The figure shows three views and two pictorial views of one solid part (mm, origin at its lowest corner). Answer the questions. A direction names the side the tool comes from. Round coordinates to 2 decimals unless told otherwise and drop trailing zeros. Order: outer loops, then holes, each group sorted by start corner. A loop starts at its lowest first (then second) coordinate and runs counter-clockwise, first axis right, second up. Notation, with made-up numbers: (4, -22) - (48, -22) arc R35 ccw to (48, 16) - close; hole circle Ø2 at (7.25, 42.5). An arc over 180 degrees is marked (long way). One line per item, written item: value. Start each with the question number.
1. Straight lines are drawn through the part: line 1 (X direction, y = 0.4, z = 35); line 2 (Y direction, x = 41, z = 54.5); line 3 (Z direction, x = 27.5, y = 0.85). For each, find the intervals that lie inside material, in ascending order.
2. Section C-C, the plane z = 50.5 is taken. Give the vertices of the cut face in (x, y).
3. Section A-A, the plane x = 7 is taken. Give the vertices of the cut face in (y, z), then the cut area to 3 significant figures.
4. Flat-ended cylindrical pins translate along their axes: P1, Ø0.6, axis at x = 43, y = 1, coming from the -Z side; P2, Ø8, axis at x = 24, z = 48, coming from the +Y side; P3, Ø2, axis at y = 1, z = 15, coming from the +X side. Find the tip coordinate at first contact, or state that the pin passes through.
5. Section B-B, the plane y = 3.5 is taken. Give the vertices of the cut face in (x, z), then the cut area to 3 significant figures.
6. A tool of negligible diameter and unlimited length cuts with its end or side. For the marked faces 1 and 2, from which of +Z, -Z, +X, -X, +Y, -Y can it reach the whole face along a straight path? Write none if from no direction.
7. Section D-D, the plane z = 38 is taken. Give the vertices of the cut face in (x, y).
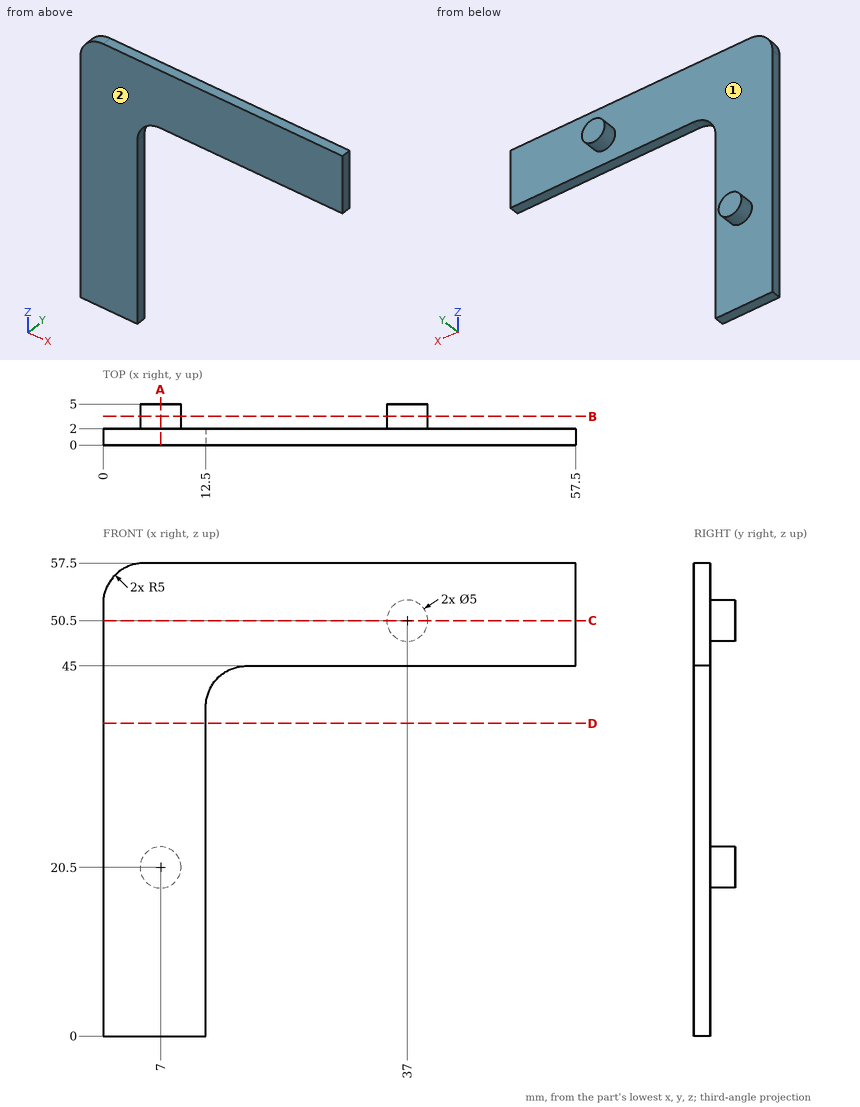
Answer list:
1. line 1: x = 0 to 12.5
1. line 2: y = 0 to 2
1. line 3: z = 45 to 57.5
2. outline: (0, 0) - (57.5, 0) - (57.5, 2) - (39.5, 2) - (39.5, 5) - (34.5, 5) - (34.5, 2) - (0, 2) - close
3. outline: (0, 0) - (2, 0) - (2, 18) - (5, 18) - (5, 23) - (2, 23) - (2, 57.5) - (0, 57.5) - close
3. area: 130 mm²
4. P1: stops at z = 45
4. P2: stops at y = 2
4. P3: stops at x = 12.5
5. outline: circle Ø5 at (7, 20.5); circle Ø5 at (37, 50.5)
5. area: 39.3 mm²
6. face 1: +Y
6. face 2: +Z, -Z, +X, -X, -Y
7. outline: (0, 0) - (12.5, 0) - (12.5, 2) - (0, 2) - close
